Can you work these out from the model? Positions are in its coordinate system, mm. Coordinates: 2 decimals unless noted, no trailing zeros. Write each loop counter-clockwise with the first axis right and the second up, starting at its lowest first coordinate (ties: lowest second). Pieces come first, ordered by that corner, then holes. Notation, with made-up numbers: (42.25, 35.5) - (78.25, 35.5) arc R30 cw to (78.25, 68.5) - close; hole circle Ø11 at (34.5, 44). An arc over 180 degrees is marked (long way). Write each question's results on one line, items separated by ' | '. Start each with the question number.
```python
from build123d import *

# Parameters (mm, degrees)
SKETCH1_R           = 2.5
BOSS_EXTRUDE1_DEPTH = 3


with BuildPart() as part:
    # Sketch1 → Boss-Extrude1 (new body)
    with BuildSketch(Plane.XY):
        with BuildLine():
            Line((10.853563951, -84.90575827), (-10.853563951, -84.90575827))
            Line((-10.853563951, -84.90575827), (-4.782100014, 10.606475312))
            ThreePointArc((-4.782100014, 10.606475312), (-3.279044371, 13.796592676), (0, 15.09424173))
            ThreePointArc((0, 15.09424173), (3.279044371, 13.796592676), (4.782100014, 10.606475312))
            Line((4.782100014, 10.606475312), (10.853563951, -84.90575827))
        make_face()
        with Locations((0, 10.09424173)):
            Circle(SKETCH1_R, mode=Mode.SUBTRACT)
    extrude(amount=BOSS_EXTRUDE1_DEPTH)


solid = part.part
```
Q1. Thinking about a two-plate mould opening in X: for faces 1 (the face through (-0.325, 12.573, 1.479)), 2 (the face through (-7.86, -37.82, 1.48)), 3 (the face through (0, -84.906, 1)), which applies, pulls with the +X half, pulls with the -X half, needs draft (parallel to the pull), parting line crosses it, or undercut?
Q2. If we section it at C-C (x = -9): Please give me the cut outline in (y, z).
Q3. If we section it at A-A (z = 0.95): Please give me the cut outline in (x, y).
Q4. I'm going to push a flat-ended pin straight in: pin 1 Ø1 at (y, z) = (-40, 1.5) entering from -X. Where does the tip first touch, or does it pass through?
Q5. I need wall thicknesses on line 1 along Y through (x, z) = (1.75, 0.3); line 2 along Y through (x, z) = (-0.5, 0.55); line 3 along X through (y, z) = (9.5, 1.95). Which ranges of each line are inside material? Lowest first, please. Write a range as from..to.
Q6. If we section it at B-B (y = -6): Please give me the cut outline in (x, z), then the cut area to 3 significant figures.
Answer list:
1) face 1: undercut | face 2: pulls with the -X half | face 3: needs draft
2) outline: (-84.91, 0) - (-55.75, 0) - (-55.75, 3) - (-84.91, 3) - close
3) outline: (-10.85, -84.91) - (10.85, -84.91) - (4.78, 10.61) arc R4.79 ccw to (-4.78, 10.61) - close; hole circle Ø5 at (0, 10.09)
4) pin 1: stops at x = -8.03
5) line 1: y = -84.91..8.31, 11.88..14.76 | line 2: y = -84.91..7.64, 12.54..15.07 | line 3: x = -4.85..-2.43, 2.43..4.85
6) outline: (-5.84, 0) - (5.84, 0) - (5.84, 3) - (-5.84, 3) - close | area: 35.0 mm2
